Model file for the job. Use its own axes, mm. A direction names the side the tool comes from. Round coordinates to 2 decimals unless told otherwise and drop trailing zeros. Loops run counter-clockwise (first coordinate to the right, second up) from the corner with the lowest first, then second, coordinate; pieces in that order, holes last. Notation, with made-up numbers: (41.5, -7.75) -> (96.5, -7.75) arc R10 cw to (96.5, -0.75) -> close; hole circle Ø3 at (36.5, -28). An arc over 180 degrees is marked (long way). Use a Markdown table: item, result. Add a question column.
```python
from build123d import *

# Parameters (mm, degrees)
F0_R     = 11
F1_DEPTH = 2
F2_R     = 5
F3_DEPTH = 1
F4_R     = 4
F5_DEPTH = 3


with BuildPart() as f1:
    # F0 (on Top) → F1 (new body)
    with BuildSketch(Plane.XY):
        Circle(F0_R)
    extrude(amount=F1_DEPTH)

    # F2 (on face) → F3 (join)
    with BuildSketch(Plane.XY.offset(2)):
        Circle(F2_R)
    extrude(amount=F3_DEPTH)

    # F4 (on face) → F5 (join)
    with BuildSketch(Plane.XY.offset(3)):
        Circle(F4_R)
    extrude(amount=F5_DEPTH)


solid = f1.part
```
1) Pin check, flat tips, straight feed: pin 1 Ø1 at (x, y) = (-6.5, 1) entering from -Z; pin 2 Ø1.5 at (x, z) = (-5, 4.5) entering from +Y. Stop position of each tip, or through.
2) Tool access for faces 1 (the face through (0, 0, 6)), 2 (the face through (-1.08, -4.88, 2.49)): list every direction of +Z, -Z, +X, -X, +Y, -Y with a clear straight run to the whole face (end or side of a thin tool).
3) Cut at A-A on x = 0. Write the cut outline in (y, z).
4) Cut at D-D on y = -4.5. Write the cut outline in (x, z).
5) Wall check: probe 1 along Z at (x, y) = (-3, -9.75); probe 2 along Y at (x, z) = (-1.25, 4.9); probe 3 along X at (y, z) = (-3.5, 3.1). Give the ranges that are in metal, low to high. Write a range as from..to.
6) Pull direction Z, two halves, no side cores. Call faces 3 (the face through (2, -5, 2)), 4 (the face through (-2.38, -10.74, 0.99)), 5 (the face through (0, 0, 0)): +Z half, -Z half, draft (parallel to the pull), parting line (faces both ways), or undercut.
7) Cut at C-C on z = 3.4. Write the cut outline in (x, y).
Established:
| question | item | result |
|---|---|---|
| 1 | pin 1 | stops at z = 0 |
| 1 | pin 2 | passes through |
| 2 | face 1 | +Z, +X, -X, +Y, -Y |
| 2 | face 2 | +Z |
| 3 | outline | (-11, 0) -> (11, 0) -> (11, 2) -> (5, 2) -> (5, 3) -> (4, 3) -> (4, 6) -> (-4, 6) -> (-4, 3) -> (-5, 3) -> (-5, 2) -> (-11, 2) -> close |
| 4 | outline | (-10.04, 0) -> (10.04, 0) -> (10.04, 2) -> (2.18, 2) -> (2.18, 3) -> (-2.18, 3) -> (-2.18, 2) -> (-10.04, 2) -> close |
| 5 | probe 1 | z = 0..2 |
| 5 | probe 2 | y = -3.8..3.8 |
| 5 | probe 3 | x = -1.94..1.94 |
| 6 | face 3 | +Z half |
| 6 | face 4 | draft |
| 6 | face 5 | -Z half |
| 7 | outline | circle Ø8 at (0, 0) |
